Geometry check sheet. Reference: the model listing, model coordinates, mm. Face numbers are marked on the shaded views. A direction names the side the tool comes from. Round coordinates to 2 decimals unless told otherwise and drop trailing zeros. Order: outer loops, then holes, each group sorted by start corner. A loop starts at its lowest first (then second) coordinate and runs counter-clockwise, first axis right, second up.
(1) Material ranges on line 1 along X through (y, z) = (-2, 0); line 2 along Y through (x, z) = (-14, 3); line 3 along Y through (x, z) = (-4, -9.5), recorded low to high.
(2) Sectioned sample at B-B (z = 0). Give the number of separate pieces and of enclosed holes in the cut face, plus the area to 3 significant figures.
(3) Set-up check for the marked faces 5, 6, 7, 8 and 9: record each of +Z, -Z, +X, -X, +Y, -Y from which the full face is reachable in a straight line by a thin tool's end or side.
(4) Go/stop test with flat-tipped pins: pin 1 (8 mm diameter, centred on y = -35.5, z = -3, fed in from +X) (3 decimals); pin 2 (15 mm diameter, centred on x = -8, z = -7.5, fed in from -Y); pin 3 (4 mm diameter, centred on x = -13.5, y = -6, fed in from -Z); pin 4 (16 mm diameter, centred on x = -6, z = -3.5, fed in from +Y). Record where each tip stops, or that it passes through.
(5) Sectioned sample at D-D (y = -17). Record the boundary of the cut face in (x, z) (3 decimals).
(6) Sectioned sample at A-A (y = -1.5). Record the boundary of the cut face in (x, z).
(7) Release check for a two-part mould opening along Z. For the marked faces 1, 2, 3 and 4 record: +Z half, -Z half, draft (parallel to the pull), parting line (faces both ways), or undercut.
from build123d import *

# Parameters (mm, degrees)
BOSS_EXTRUDE1_DEPTH      = 6
BOSS_EXTRUDE1_DEPTH_BACK = 49.9
SKETCH2_R                = 2.65
SKETCH3_R                = 1.78
CUT_EXTRUDE1_DEPTH       = 6
SKETCH4_W                = 5.711822604
SKETCH4_H                = 7.4
CUT_EXTRUDE2_DEPTH       = 60.035942442
CHAMFER1_SIZE            = 0.2


with BuildPart() as part:
    # Sketch1 → Revolve1 (revolve)
    with BuildSketch(Plane.XY, mode=Mode.PRIVATE) as revolve1_sk:
        Polygon((0, 3.05), (-15.875, 3.05), (-15.875, 0), (-25.4, 0), (-25.4, -3.05), (-15.875, -3.05), (-15.875, -13.05), (-14.875, -13.05), (-14.875, -15.05), (-15.875, -15.05), (-15.875, -27.45), (-14.875, -27.45), (-14.875, -27.95), (-15.875, -27.95), (-15.875, -40.85), (0, -40.85), align=None)
    revolve(revolve1_sk.sketch.rotate(Axis((0, 50.719281348, 0), (0, -1, 0)), 270), axis=Axis((0, 50.719281348, 0), (0, -1, 0)))

    # Sketch2 → Boss-Extrude1 (add, two sides: drawn at the far end of the back side and taken through both)
    with BuildSketch(Plane(origin=(0, 3.05, 0), x_dir=(1, 0, 0), z_dir=(0, 1, 0)).offset(-BOSS_EXTRUDE1_DEPTH_BACK)):
        with Locations(Location((0, 0, 0), (0, 0, 270))):
            Circle(SKETCH2_R)
        with Locations(Location((0, -10.5, 0), (0, 0, 270))):
            Circle(SKETCH2_R)
    extrude(amount=BOSS_EXTRUDE1_DEPTH + BOSS_EXTRUDE1_DEPTH_BACK)

    # Sketch3 → Cut-Extrude1 (cut)
    with BuildSketch(Plane(origin=(0, 0, 0), x_dir=(1, 0, 0), z_dir=(0, 1, 0))):
        with Locations(Location((0, 20.64, 0), (0, 0, 270))):
            Circle(SKETCH3_R)
        with Locations(Location((-20.64, 0, 0), (0, 0, 270))):
            Circle(SKETCH3_R)
        with Locations(Location((0, -20.64, 0), (0, 0, 270))):
            Circle(SKETCH3_R)
        with Locations(Location((20.64, 0, 0), (0, 0, 270))):
            Circle(SKETCH3_R)
    extrude(amount=-CUT_EXTRUDE1_DEPTH, mode=Mode.SUBTRACT)

    # Sketch4 → Cut-Extrude2 (cut, symmetric)
    with BuildSketch(Plane.XY):
        with Locations((-15.935911302, -9.35)):
            Rectangle(SKETCH4_W, SKETCH4_H)
        with Locations((-15.935911302, -37.184964336)):
            Rectangle(SKETCH4_W, SKETCH4_H)
    cut_extrude2 = extrude(amount=CUT_EXTRUDE2_DEPTH, both=True, mode=Mode.SUBTRACT)

    # Mirror1: Cut-Extrude2 across plane
    add(cut_extrude2.mirror(Plane(origin=(0, 0, 0), x_dir=(0, 0, 1), z_dir=(1, 0, 0))), mode=Mode.SUBTRACT)

    # Chamfer1
    chamfer1_edges = [part.edges().sort_by_distance(p)[0] for p in [
        (13.08, -40.85, 0),
        (0, -13.05, -15.875),
        (0, -3.05, -25.4),
        (0, 0, -25.4),
        (0, -46.85, -2.65),
        (0, 9.05, -2.65),
        (0, -46.85, 7.85),
        (0, 9.05, 7.85),
        (-13.08, -40.85, 0),
        (-7.389284751, -13.05, 14.050412658),
    ]]
    chamfer(chamfer1_edges, length=CHAMFER1_SIZE)


solid = part.part
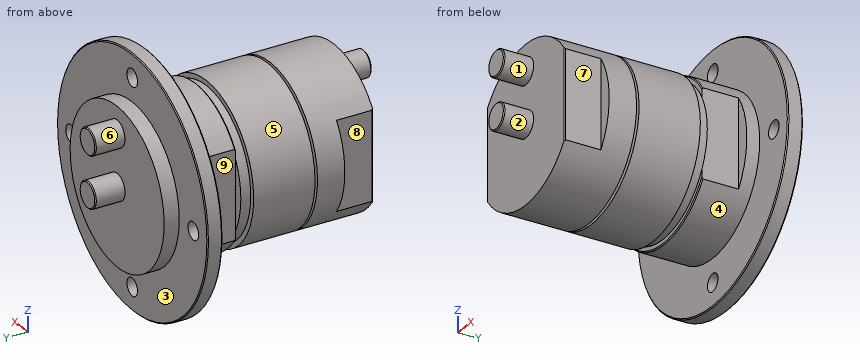
Answer below:
1. line 1: x = -25.4 to -22.42, -18.86 to 18.86, 22.42 to 25.4
1. line 2: y = -33.48 to -13.05, -5.65 to 3.05
1. line 3: y = -40.85 to 3.05
2. separate pieces: 3
2. enclosed holes: 0
2. area: 1,410 mm2
3. face 5: -Y
3. face 6: +Y
3. face 7: +Z, -Z, +X, -Y
3. face 8: +Z, -Z, -X, -Y
3. face 9: +Z, -Z, -X
4. pin 1: stops at x = 15.875
4. pin 2: stops at y = -40.85
4. pin 3: stops at z = -10.94
4. pin 4: stops at y = 9.05
5. outline: circle Ø31.75 at (0, 0)
6. outline: circle Ø50.8 at (0, 0); hole circle Ø3.56 at (-20.64, 0); hole circle Ø3.56 at (0, -20.64); hole circle Ø3.56 at (0, 20.64); hole circle Ø3.56 at (20.64, 0)
7. face 1: undercut
7. face 2: undercut
7. face 3: draft
7. face 4: parting line
